Could you check a few things on this drawing? It's one solid part, dimensions in mm from its lowest x, y, z. A direction names the side the tool comes from. Give positions to 0.01 mm unless a question says otherwise; leave off trailing zeros. Order: outer loops, then holes, each group sorted by start corner. A loop starts at its lowest first (then second) coordinate and runs counter-clockwise, first axis right, second up.
(1) Will these pins go through, and if not, where does the flat tip stop? pin 1 (8 mm diameter, centred on x = 36, y = 18.5, fed in from +Z); pin 2 (2 mm diameter, centred on x = 0.5, y = 17.5, fed in from +Z); pin 3 (2.5 mm diameter, centred on x = 33.5, y = 7, fed in from +Z); pin 4 (2.5 mm diameter, centred on x = 40.5, y = 14.5, fed in from +Z).
(2) Imagine slicing it at D-D, the plane z = 25. Write out the boundary of the cut face in (x, y).
(3) Imagine slicing it at C-C, the plane y = 13.25. Write out the boundary of the cut face in (x, z), then the cut area to 3 significant figures.
(4) Imagine slicing it at A-A, the plane y = 19.25. Write out the boundary of the cut face in (x, z).
(5) If we mould it in two halves opening along Z, with no side actions, what happens to the marked faces 5, 6 and 7? For each: released by +Z, released by -Z, zero draft, split by the parting line, or undercut.
(6) Imagine slicing it at B-B, the plane x = 14. Write out the boundary of the cut face in (y, z).
(7) On a 3-axis mill with a long thin cutter (end or side, diameter ignored), from which of +Z, -Z, +X, -X, +Y, -Y can I reach the whole of each face in a straight line? I mean the marked faces 1, 2, 3 and 4. Say none if no direction works.
(8) If I drill on probe 1 along X at (y, z) = (20, 34); probe 2 along Y at (x, z) = (11.5, 10.5); probe 3 along Z at (x, y) = (16, 4.75) (1 decimal), over which ranges is the centre line in solid material (lowest first)?
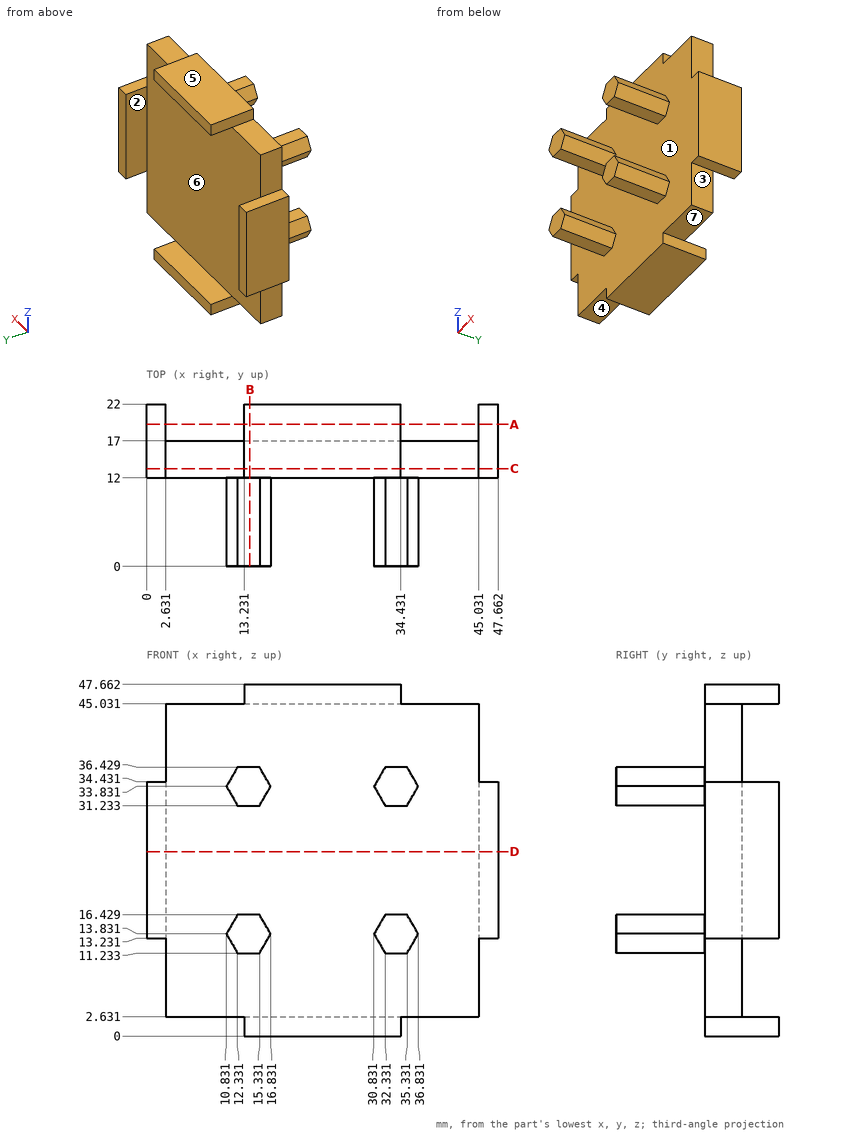
Answer block:
1. pin 1: stops at z = 47.66
1. pin 2: stops at z = 34.43
1. pin 3: stops at z = 36.43
1. pin 4: stops at z = 45.03
2. outline: (0, 12) - (47.66, 12) - (47.66, 22) - (45.03, 22) - (45.03, 17) - (2.63, 17) - (2.63, 22) - (0, 22) - close
3. outline: (0, 13.23) - (2.63, 13.23) - (2.63, 2.63) - (13.23, 2.63) - (13.23, 0) - (34.43, 0) - (34.43, 2.63) - (45.03, 2.63) - (45.03, 13.23) - (47.66, 13.23) - (47.66, 34.43) - (45.03, 34.43) - (45.03, 45.03) - (34.43, 45.03) - (34.43, 47.66) - (13.23, 47.66) - (13.23, 45.03) - (2.63, 45.03) - (2.63, 34.43) - (0, 34.43) - close
3. area: 2,020 mm2
4. outline: (0, 13.23) - (2.63, 13.23) - (2.63, 34.43) - (0, 34.43) - close; (13.23, 0) - (34.43, 0) - (34.43, 2.63) - (13.23, 2.63) - close; (13.23, 45.03) - (34.43, 45.03) - (34.43, 47.66) - (13.23, 47.66) - close; (45.03, 13.23) - (47.66, 13.23) - (47.66, 34.43) - (45.03, 34.43) - close
5. face 5: released by +Z
5. face 6: undercut
5. face 7: released by -Z
6. outline: (0, 11.23) - (12, 11.23) - (12, 0) - (22, 0) - (22, 2.63) - (17, 2.63) - (17, 45.03) - (22, 45.03) - (22, 47.66) - (12, 47.66) - (12, 36.43) - (0, 36.43) - (0, 31.23) - (12, 31.23) - (12, 16.43) - (0, 16.43) - close
7. face 1: -Y
7. face 2: +Z, -Z, +Y
7. face 3: -Z, +X, +Y, -Y
7. face 4: -Z, -X, +Y, -Y
8. probe 1: x = 0 to 2.63, 45.03 to 47.66
8. probe 2: y = 12 to 17
8. probe 3: z = 12.4 to 15.3, 32.4 to 35.3
